Input: dimensioned drawing with shaded views. Units: mm. Origin: part minimum x, y, z. A direction names the side the tool comes from. Round coordinates to 2 decimals unless told otherwise and drop trailing zeros. Write each loop counter-clockwise with the first axis right and the second up, starting at its lowest first coordinate (ties: lowest second). Pieces come first, ordered by that corner, then holes. Notation, with made-up numbers: M -29,74.5 L 11,74.5 A16 cw 11,94.5 Z; hole C 19.25,84.25 d1. An arc over 180 degrees is marked long. Use one line per item in the form item = value. Start each with the question number.
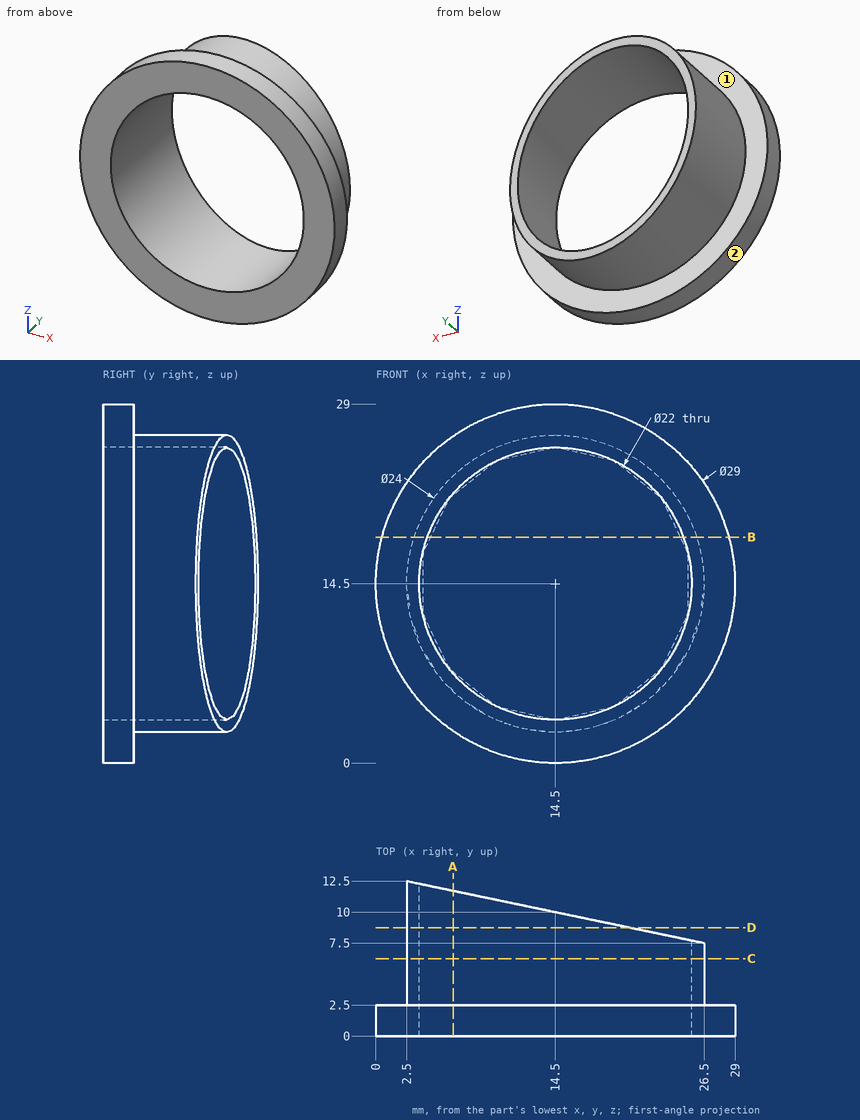
1. Contact query for flat-ended pins moving along their axis: pin 1 (1.5 mm diameter, centred on y = 1.5, z = 17.5, fed in from +X); pin 2 (2 mm diameter, centred on y = 6.5, z = 13, fed in from +X); pin 3 (3 mm diameter, centred on x = 12, z = 24, fed in from +Y). Output: stop coordinate, or through.
2. Ray query, probe 1 along Z at (x, y) = (14.5, 5.5); probe 2 along Z at (x, y) = (9.25, 10.25). Return the intervals inside material, ascending.
3. Section query D-D (y = 8.75). Return loops of the section in (x, z).
4. Set-up query: the marked faces 1 and 2. Return all of +Z, -Z, +X, -X, +Y, -Y with unobstructed straight access to the full face (end or side cutting, diameter ignored); none if empty.
5. Section query A-A (x = 6.25). Return loops of the section in (y, z).
6. Section query C-C (y = 6.25). Return loops of the section in (x, z).
7. Section query B-B (z = 18.25). Return loops of the section in (x, y).
Checks:
q1.pin_1 = 28.82
q1.pin_2 = 26.49
q1.pin_3 = 10.78
q2.probe_1 = 2.5 to 3.5, 25.5 to 26.5
q2.probe_2 = 3.71 to 4.83, 24.17 to 25.29
q3.outline = M 20.5,4.11 L 20.5,5.28 A11 cw long 20.5,23.72 L 20.5,24.89 A12 ccw long Z
q4.face_1 = +Y
q4.face_2 = +Y, -Y
q5.outline = M 0,2.58 L 2.5,2.58 L 2.5,5.79 L 11.72,5.79 L 11.72,7.22 L 0,7.22 Z; M 0,21.78 L 11.72,21.78 L 11.72,23.21 L 2.5,23.21 L 2.5,26.42 L 0,26.42 Z
q6.outline = C 14.5,14.5 d24; hole C 14.5,14.5 d22
q7.outline = M 0.49,0 L 4.16,0 L 4.16,12.15 L 3.1,12.37 L 3.1,2.5 L 0.49,2.5 Z; M 24.84,0 L 28.51,0 L 28.51,2.5 L 25.9,2.5 L 25.9,7.63 L 24.84,7.85 Z
